Part model, mm, in its own coordinate system. Round coordinates to 2 decimals unless told otherwise and drop trailing zeros. Write each loop counter-clockwise with the first axis right and the second up, starting at its lowest first coordinate (ties: lowest second). Pieces come first, ordered by that corner, then holes. Notation, with made-up numbers: M 8.5,52 L 67.5,52 A34 ccw 67.5,84 Z; hole C 65,71.5 d7. An arc over 180 degrees is marked long. Answer as a JSON object with one key per item and string values. Group by question number.
1. Band-saw the part on C-C, the plane y = 10. Write the cut outline in (x, z), plus the area to 3 significant figures.
2. Drop a flat-ended pin along its axis: pin 1 (3 mm diameter, centred on x = 10, z = 5, fed in from -Y). Give the stop position or say it passes through.
3. Band-saw the part on A-A, the plane z = 5. Write the cut outline in (x, y).
4. Band-saw the part on B-B, the plane x = 70. Write the cut outline in (y, z).
5. Drill centre lines: line 1 (X direction, y = 4, z = 5); line 2 (Z direction, x = 70, y = 2.5); line 3 (X direction, y = 0.75, z = 4.25). Where is each one in solid material? Low to high. Write a range as from..to.
from build123d import *

# Parameters (mm, degrees)
SKETCH_1_W          = 80
SKETCH_1_H          = 12
EXTRUDE_1_DEPTH     = 11.5
CUT_EXTRUDE_1_REACH = 83.708
SKETCH_2_R          = 1.55
SKETCH_3_W          = 80
SKETCH_3_H          = 12
CUT_EXTRUDE_2_DEPTH = 0.2


with BuildPart() as part:
    # 草图1 → 凸台-拉伸1 (new body)
    with BuildSketch(Plane.XY):
        with Locations((40, 6)):
            Rectangle(SKETCH_1_W, SKETCH_1_H)
    extrude(amount=EXTRUDE_1_DEPTH)

    # 草图2 → 切除-拉伸1 (cut, up to next)
    with BuildSketch(Plane(origin=(0, 12, 0), x_dir=(1, 0, 0), z_dir=(0, 1, 0)), mode=Mode.PRIVATE) as cut_extrude_1_sk1:
        with Locations(Location((10, -5, 0), (0, 0, 270))):
            Circle(SKETCH_2_R)
    cut_extrude_1_tool1 = extrude(cut_extrude_1_sk1.sketch, amount=-CUT_EXTRUDE_1_REACH, mode=Mode.PRIVATE) & part.part
    # 草图2 → 切除-拉伸1 (cut, up to next)
    with BuildSketch(Plane(origin=(0, 12, 0), x_dir=(1, 0, 0), z_dir=(0, 1, 0)), mode=Mode.PRIVATE) as cut_extrude_1_sk2:
        with Locations(Location((70, -5, 0), (0, 0, 270))):
            Circle(SKETCH_2_R)
    cut_extrude_1_tool2 = extrude(cut_extrude_1_sk2.sketch, amount=-CUT_EXTRUDE_1_REACH, mode=Mode.PRIVATE) & part.part
    add(cut_extrude_1_tool1.solids().sort_by_distance((10, 12, 5))[0], mode=Mode.SUBTRACT)
    add(cut_extrude_1_tool2.solids().sort_by_distance((70, 12, 5))[0], mode=Mode.SUBTRACT)

    # 草图3 → 切除-拉伸2 (cut)
    with BuildSketch(Plane.XY.offset(11.5)):
        with Locations((40, 6)):
            Rectangle(SKETCH_3_W, SKETCH_3_H)
    extrude(amount=-CUT_EXTRUDE_2_DEPTH, mode=Mode.SUBTRACT)


solid = part.part
Worked answers:
{
 "1": {"outline": "M 0,0 L 80,0 L 80,11.3 L 0,11.3 Z; hole C 10,5 d3.1; hole C 70,5 d3.1", "area": "889 mm^2"},
 "2": {"pin 1": "passes through"},
 "3": {"outline": "M 0,0 L 8.45,0 L 8.45,12 L 0,12 Z; M 11.55,0 L 68.45,0 L 68.45,12 L 11.55,12 Z; M 71.55,0 L 80,0 L 80,12 L 71.55,12 Z"},
 "4": {"outline": "M 0,0 L 12,0 L 12,3.45 L 0,3.45 Z; M 0,6.55 L 12,6.55 L 12,11.3 L 0,11.3 Z"},
 "5": {"line 1": "x = 0..8.45, 11.55..68.45, 71.55..80", "line 2": "z = 0..3.45, 6.55..11.3", "line 3": "x = 0..8.64, 11.36..68.64, 71.36..80"}
}
